Check sheet for the modelled part. Datum: model origin and axes. Units: mm. A direction names the side the tool comes from. Round coordinates to 2 decimals unless told otherwise and drop trailing zeros. Loops run counter-clockwise (first coordinate to the right, second up) from the corner with the lowest first, then second, coordinate; pieces in that order, holes last. Notation, with made-up numbers: (6.25, 27.5) -> (37.25, 27.5) arc R16 cw to (37.25, 39.5) -> close; hole circle Ø2 at (81.25, -29). An arc over 180 degrees is marked (long way). Return JSON: item names as keys, results as strings.
from build123d import *

# Parameters (mm, degrees)
BOSS_EXTRUDE1_DEPTH = 16
SKETCH10_R          = 8.9195787
BOSS_EXTRUDE8_DEPTH = 3.5
BOSS_EXTRUDE8_TAPER = 50
SKETCH12_R          = 2
CUT_EXTRUDE3_DEPTH  = 48.178799534
CUT_EXTRUDE4_START  = -4
SKETCH13_R          = 4.25
CUT_EXTRUDE4_DEPTH  = 44.178799534


with BuildPart() as part:
    # Sketch1 → Boss-Extrude1 (new body)
    with BuildSketch(Plane(origin=(0, 0, 0), x_dir=(1, 0, 0), z_dir=(0, 1, 0))):
        with BuildLine():
            Line((-10, 10), (10, 10))
            Line((10, 10), (10, -10))
            Line((10, -10), (12, -10))
            Line((12, -10), (34.369481018, 21.946929727))
            ThreePointArc((34.369481018, 21.946929727), (33.370084476, 33.370084476), (21.946929727, 34.369481018))
            Line((21.946929727, 34.369481018), (-10, 12))
            Line((-10, 12), (-10, 10))
        make_face()
    extrude(amount=-BOSS_EXTRUDE1_DEPTH)

    # Sketch10 → Boss-Extrude8 (add)
    with BuildSketch(Plane(origin=(0, 0, 0), x_dir=(1, 0, 0), z_dir=(0, 1, 0))):
        with Locations((27.062989892, 27.062989892)):
            Circle(SKETCH10_R)
    extrude(amount=BOSS_EXTRUDE8_DEPTH, taper=BOSS_EXTRUDE8_TAPER)

    # Sketch12 → Cut-Extrude3 (cut, through all)
    with BuildSketch(Plane.ZY.offset(-10)):
        with Locations((0, -8)):
            Circle(SKETCH12_R)
    cut_extrude3 = extrude(amount=-CUT_EXTRUDE3_DEPTH, mode=Mode.SUBTRACT)

    # Sketch13 → Cut-Extrude4 (cut, through all)
    with BuildSketch(Plane.ZY.offset(-10).offset(CUT_EXTRUDE4_START)):
        with Locations((0, -8)):
            Circle(SKETCH13_R)
    cut_extrude4 = extrude(amount=-CUT_EXTRUDE4_DEPTH, mode=Mode.SUBTRACT)

    # Mirror3: Cut-Extrude3, Cut-Extrude4 across plane
    add(cut_extrude3.mirror(Plane(origin=(0, 0, 0), x_dir=(-0.7071067811865478, 0, 0.7071067811865472), z_dir=(-0.7071067811865475, 0, -0.7071067811865477))), mode=Mode.SUBTRACT)
    add(cut_extrude4.mirror(Plane(origin=(0, 0, 0), x_dir=(-0.7071067811865478, 0, 0.7071067811865472), z_dir=(-0.7071067811865475, 0, -0.7071067811865477))), mode=Mode.SUBTRACT)


solid = part.part
Q1. Tool access check on faces 4 (the cylindrical face through (4.246, -7.813, -17.094)), 5 (the flat face through (14, -9, 2)), 6 (the flat face through (23.03, -7.89, -5.75)), 7 (the flat face through (-2.4, -7.9, -10)), 8 (the flat face through (6.197, -7.888, -23.341)). Record the directions out of +Z, -Z, +X, -X, +Y, -Y that give a thin tool (end or side, any length) a straight path to the whole face; none if there is none.
Results list:
{"face 4": "-Z", "face 5": "+X", "face 6": "+Z, +X, +Y, -Y", "face 7": "+Z, -X, +Y, -Y", "face 8": "-Z, -X, +Y, -Y"}
Q2. Go/stop test with flat-tipped pins: pin 1 (6 mm diameter, centred on y = -4.5, z = -31, fed in from +X); pin 2 (7 mm diameter, centred on x = 2, y = -7.5, fed in from -Z); pin 3 (1 mm diameter, centred on x = 14, y = -5.5, fed in from -Z). Record where each tip stops, or that it passes through.
Results list:
{"pin 1": "x = 35.93", "pin 2": "z = -22.85", "pin 3": "z = -29.16"}
Q3. Material ranges on line 1 (Y direction, x = 0, z = -12); line 2 (Y direction, x = 12.5, z = -25); line 3 (Y direction, x = 0, z = -18), recorded low to high.
Results list:
{"line 1": "-16 to -10, -6 to 0", "line 2": "-16 to 0", "line 3": "-16 to -12.25, -3.75 to 0"}
Q4. Section check B-B (z = 0). Record the boundary of the cut face in (x, y), then the cut area to 3 significant figures.
Results list:
{"outline": "(10, -16) -> (19, -16) -> (19, -12.25) -> (14, -12.25) -> (14, -10) -> (10, -10) -> close; (10, -6) -> (14, -6) -> (14, -3.75) -> (19, -3.75) -> (19, 0) -> (10, 0) -> close", "area": "85.5 mm^2"}
Q5. Section check C-C (y = -8). Record the boundary of the cut face in (x, z).
Results list:
{"outline": "(-10, -12) -> (-4.25, -16.03) -> (-4.25, -14) -> (-2, -14) -> (-2, -10) -> (-10, -10) -> close; (2, -14) -> (4.25, -14) -> (4.25, -21.98) -> (21.95, -34.37) arc R8.92 ccw to (34.37, -21.95) -> (21.98, -4.25) -> (14, -4.25) -> (14, -2) -> (10, -2) -> (10, -10) -> (2, -10) -> close; (10, 2) -> (14, 2) -> (14, 4.25) -> (16.03, 4.25) -> (12, 10) -> (10, 10) -> close"}
Q6. Draft check along Y on faces 1 (the flat face through (-2, -9, -14)), 2 (the flat face through (12, 0, -14)), 3 (the cylindrical face through (33.49, -7.89, -33.25)). Enter one of: released by +Y, released by -Y, zero draft, split by the parting line, or undercut.
Results list:
{"face 1": "undercut", "face 2": "released by +Y", "face 3": "zero draft"}
Q7. Section check D-D (z = -13). Record the boundary of the cut face in (x, y).
Results list:
{"outline": "(-8.57, -16) -> (28.1, -16) -> (28.1, 0) -> (-8.57, 0) -> close; hole circle Ø4 at (0, -8)"}
Q8. Section check A-A (x = 0). Record the boundary of the cut face in (y, z), then the cut area to 3 significant figures.
Results list:
{"outline": "(-16, -19) -> (-12.25, -19) -> (-12.25, -14) -> (-10, -14) -> (-10, -10) -> (-16, -10) -> close; (-6, -14) -> (-3.75, -14) -> (-3.75, -19) -> (0, -19) -> (0, -10) -> (-6, -10) -> close", "area": "85.5 mm^2"}
